Read the model definition and answer for the solid it produces. Units are mm, in the model's axes. Face numbers are marked on the shaded views. A direction names the side the tool comes from. Give positions to 0.01 mm unless a question says otherwise; leave off trailing zeros. Order: outer loops, then holes, each group sorted by start corner. A loop starts at its lowest first (then second) coordinate and runs counter-clockwise, first axis right, second up.
Item 1: Given pin 1 Ø2 at (x, y) = (-20.5, 5) entering from -Z; pin 2 Ø1.5 at (x, y) = (-18, 8) entering from -Z; pin 3 Ø1 at (x, y) = (-2.5, 1.5) entering from -Z; pin 4 Ø4 at (y, z) = (5, -20.5) entering from -X, each flat-ended and moving along its own axis, determine where each tip first touches the part or whether it passes through.
Item 2: A cutting plane is placed at C-C (y = 4.25). State how many separate pieces and enclosed holes the cut face has, plus the area to 3 significant figures.
Item 3: A cutting plane is placed at A-A (x = -20.5). Write down the section's boundary in (y, z), plus the area to 3 significant figures.
Item 4: Which of the six approach directions +Z, -Z, +X, -X, +Y, -Y give full straight-line access (tool end or side, diameter ignored) to the marked faces 4, 5 and 6?
Item 5: Find the intervals of material crossed by line 1 along Y through (x, z) = (-20.5, -0.6); line 2 along Z through (x, y) = (-15.25, 2.75), in increasing order.
Item 6: A cutting plane is placed at B-B (z = -20.5). Write down the section's boundary in (x, y).
Item 7: The mould has two halves that part along Z. Classify the marked faces 1, 2 and 3: +Z half, -Z half, draft (parallel to the pull), parting line (faces both ways), or undercut.
Autodesk Inventor part; units mm, degrees
ref_plane "YZ Plane" through (0, 0, 0) normal (1, 0, 0) x (0, 1, 0)
ref_plane "XZ Plane" through (0, 0, 0) normal (0, 1, 0) x (-1, 0, 0)
ref_plane "XY Plane" through (0, 0, 0) normal (0, 0, 1) x (1, 0, 0)
sketch "Sketch1" plane through (0, 0, 0) normal (1, 0, 0) x (0, 1, 0)
  line L0 (0, 0) -> (10, 0)
  line L1 (10, 0) -> (10, -26)
  line L2 (10, -26) -> (0, -26)
  line L3 (0, -26) -> (0, 0)
  dimension "d0" = 10
  dimension "d1" = 26
extrude "Extrusion1" add sketch "Sketch1" against normal blind 4
sketch "Sketch2" plane through (0, 0, 0) normal (0, 0, 1) x (1, 0, 0)
  line L0 (0, 0) -> (-4, 0)
  line L1 (0, 0) -> (-26, 0)
  line L2 (-26, 0) -> (-26, 10)
  line L3 (-26, 10) -> (0, 10)
  line L4 (0, 10) -> (0, 0)
  line L5 (0, 10) -> (0, 0)
  point P0 (-4, 0)
  dimension "d4" = 26
extrude "Extrusion2" add sketch "Sketch2" against normal blind 4
sketch "Sketch3" plane through (-4, 0, 0) normal (-1, 0, 0) x (0, 0, 1)
  line L0 (-18.8546, 2.15) -> (-22.1454, 2.15)
  line L1 (-22.1454, 2.15) -> (-23.7909, 5)
  line L2 (-23.7909, 5) -> (-22.1454, 7.85)
  line L3 (-22.1454, 7.85) -> (-18.8546, 7.85)
  line L4 (-18.8546, 7.85) -> (-17.2091, 5)
  line L5 (-17.2091, 5) -> (-18.8546, 2.15)
  line L6 (-26, 10) -> (-26, 0)
  point P0 (0, 0)
  point P1 (-20.5, 5)
  point P2 (-26, 5)
  dimension "d7" = 5.7
  dimension "d8" = 5.5
extrude "Extrusion3" cut sketch "Sketch3" against normal blind 2.4
sketch "Sketch4" plane through (-1.6, 0, 0) normal (-1, 0, 0) x (0, 0, 1)
  line L0 (-18.8546, 7.85) -> (-17.2091, 5)
  line L1 (-22.1454, 7.85) -> (-18.8546, 7.85)
  line L2 (-23.7909, 5) -> (-22.1454, 7.85)
  line L3 (-22.1454, 2.15) -> (-23.7909, 5)
  line L4 (-18.8546, 2.15) -> (-22.1454, 2.15)
  line L5 (-17.2091, 5) -> (-18.8546, 2.15)
  circle A0 centre (-20.5, 5) radius 1.7
  point P0 (0, 0)
  dimension "d11" = 3.4
extrude "Extrusion4" cut sketch "Sketch4" against normal up to surface (1.6 mm away) contours A0
sketch "Sketch5" plane through (0, 0, -4) normal (0, 0, -1) x (-1, 0, 0)
  line L0 (22.1454, 2.15) -> (18.8546, 2.15)
  line L1 (18.8546, 2.15) -> (17.2091, 5)
  line L2 (17.2091, 5) -> (18.8546, 7.85)
  line L3 (18.8546, 7.85) -> (22.1454, 7.85)
  line L4 (22.1454, 7.85) -> (23.7909, 5)
  line L5 (23.7909, 5) -> (22.1454, 2.15)
  line L6 (26, 0) -> (26, 10)
  point P0 (0, 0)
  point P1 (20.5, 5)
  point P2 (26, 5)
  dimension "d14" = 5.7
  dimension "d15" = 5.5
extrude "Extrusion5" cut sketch "Sketch5" against normal blind 2.4
sketch "Sketch6" plane through (0, 0, -1.6) normal (0, 0, -1) x (-1, 0, 0)
  circle A0 centre (20.5, 5) radius 1.7
  point P0 (0, 0)
  dimension "d18" = 3.4
extrude "Extrusion6" cut sketch "Sketch6" against normal up to surface (1.6 mm away)
fillet "Fillet1" radius 5 4 edges at (-2, 10, -26) (-2, 0, -26) (-26, 10, -2) (-26, 0, -2)
fillet "Fillet2" radius 5 1 edges at (-4, 5, -4)
fillet "Fillet3" radius 0.5 13 edges at (-4, 10, -15.0003) (-4, 8.5357, -24.5357) (-4, 0, -15.0003) (-5.4645, 0, -5.4645) (-24.5357, 8.5357, -4) (-15.0002, 10, -4) (-5.4645, 10, -5.4645) (0, 8.5357, -24.5357) (0, 0, -10.5003) (0, 10, -10.5003) (-24.5357, 8.5357, 0) (-10.5002, 0, 0) (-10.5002, 10, 0)
chamfer "Chamfer1" distance 0.25 angle 45 2 edges at (0, 5, -22.2) (-18.8, 5, 0)
properties part number "BoxBracket"
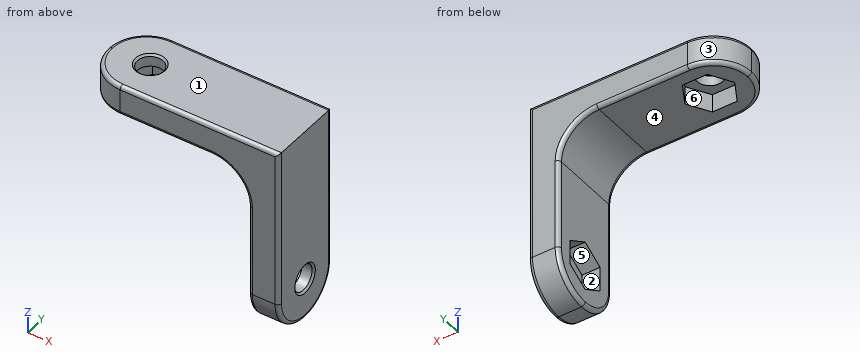
Response values:
1. pin 1: passes through
1. pin 2: stops at z = -4
1. pin 3: stops at z = -25
1. pin 4: stops at x = -1.6
2. separate pieces: 3
2. enclosed holes: 0
2. area: 159 mm2
3. outline: (0, -3.5) arc R0.5 ccw to (0.5, -4) - (2.15, -4) - (2.15, -1.6) - (3.3, -1.6) - (3.3, -0.25) - (3.05, 0) - (0.5, 0) arc R0.5 ccw to (0, -0.5) - close; (6.7, -1.6) - (7.85, -1.6) - (7.85, -4) - (9.5, -4) arc R0.5 ccw to (10, -3.5) - (10, -0.5) arc R0.5 ccw to (9.5, 0) - (6.95, 0) - (6.7, -0.25) - close
3. area: 20.6 mm2
4. face 4: -Z, -X, +Y, -Y
4. face 5: -X
4. face 6: -Z
5. line 1: y = 0 to 3.3, 6.7 to 10
5. line 2: z = -4 to 0
6. outline: (-4, 0.5) arc R0.5 ccw to (-3.5, 0) - (-0.5, 0) arc R0.5 ccw to (0, 0.5) - (0, 3.05) - (-0.25, 3.3) - (-1.6, 3.3) - (-1.6, 2.15) - (-4, 2.15) - close; (-4, 7.85) - (-1.6, 7.85) - (-1.6, 6.7) - (-0.25, 6.7) - (0, 6.95) - (0, 9.5) arc R0.5 ccw to (-0.5, 10) - (-3.5, 10) arc R0.5 ccw to (-4, 9.5) - close
7. face 1: +Z half
7. face 2: undercut
7. face 3: draft
